The listing builds one solid part. Answer for the finished solid, in the listing's coordinates (mm). A direction names the side the tool comes from. Give positions to 0.01 mm unless a question says otherwise; leave off trailing zeros. Order: outer loops, then holes, each group sorted by start corner. A loop starts at its lowest first (then second) coordinate and runs counter-clockwise, first axis right, second up. Notation, with made-up numbers: (80, 11) - (93, 11) arc R12 cw to (93, 17) - close; hole circle Ø2 at (83.25, 16.25). An arc over 180 degrees is marked (long way). Answer in a Markdown table with one row per item. Add a question column.
Autodesk Fusion 360 part; units mm, degrees
sketch "Sketch1" plane through (0, 0, 0) normal (0, 0, 1) x (1, 0, 0)
  circle A0 centre (10, 10) radius 2.5
  line L0 (13.9, 6.1) -> (6.1, 13.9) construction
  line L1 (0, 6.4) -> (0, 1.5)
  line L2 (4.5, 1.8) -> (6.9, 1.8)
  line L3 (3.5808, 4.5) -> (6.1, 7.0192)
  line L4 (4.5, 3.5808) -> (7.0192, 6.1)
  line L5 (0.5, 6.9) -> (0.5, 6.4)
  line L6 (0.5, 6.4) -> (0, 6.4)
  line L7 (6.9, 0) -> (6.4, 0) construction
  line L8 (6.4, 0) -> (6.4, 0.5)
  line L9 (6.4, 0.5) -> (6.9, 0.5)
  arc A1 (0, 1.5) -> (1.5, 0) centre (1.5, 1.5) ccw
  line L10 (1.8, 6.9) -> (0.5, 6.9)
  line L11 (1.8, 6.9) -> (1.8, 6.4)
  line L12 (1.8, 6.4) -> (1.8, 4.5)
  line L13 (3.5808, 4.5) -> (1.8, 4.5)
  line L14 (6.1, 10) -> (6.1, 7.0192)
  line L15 (7.0192, 6.1) -> (10, 6.1)
  line L16 (4.5, 1.8) -> (4.5, 3.5808)
  line L17 (6.9, 0.5) -> (6.9, 1.8)
  line L18 (1.5, 0) -> (6.4, 0)
  line L19 (6.4, 0) -> (6.9, 0)
  line L20 (0, 6.9) -> (0, 6.4)
  line L21 (10, 13.9) -> (10, 6.1) construction
  line L22 (13.9, 10) -> (6.1, 10) construction
  line L23 (20, 6.4) -> (19.5, 6.4)
  line L24 (19.5, 6.4) -> (19.5, 6.9)
  line L25 (19.5, 6.9) -> (18.2, 6.9)
  line L26 (18.2, 4.5) -> (18.2, 6.9)
  line L27 (18.2, 4.5) -> (16.4192, 4.5)
  line L28 (16.4192, 4.5) -> (13.9, 7.0192)
  line L29 (13.9, 7.0192) -> (13.9, 10)
  line L30 (15.5, 3.5808) -> (12.9808, 6.1)
  line L31 (15.5, 3.5808) -> (15.5, 1.8)
  line L32 (13.6, 1.8) -> (15.5, 1.8)
  line L33 (13.1, 1.8) -> (13.6, 1.8)
  line L34 (13.1, 1.8) -> (13.1, 0.5)
  line L35 (13.1, 0.5) -> (13.6, 0.5)
  line L36 (13.6, 0.5) -> (13.6, 0)
  line L37 (10, 6.1) -> (12.9808, 6.1)
  line L38 (13.6, 0) -> (18.5, 0)
  arc A2 (18.5, 0) -> (20, 1.5) centre (18.5, 1.5) ccw
  line L39 (20, 1.5) -> (20, 6.4)
  line L40 (13.6, 20) -> (13.6, 19.5)
  line L41 (13.6, 19.5) -> (13.1, 19.5)
  line L42 (13.1, 19.5) -> (13.1, 18.2)
  line L43 (15.5, 18.2) -> (13.1, 18.2)
  line L44 (15.5, 18.2) -> (15.5, 16.4192)
  line L45 (15.5, 16.4192) -> (12.9808, 13.9)
  line L46 (12.9808, 13.9) -> (10, 13.9)
  line L47 (16.4192, 15.5) -> (13.9, 12.9808)
  line L48 (16.4192, 15.5) -> (18.2, 15.5)
  line L49 (18.2, 13.6) -> (18.2, 15.5)
  line L50 (18.2, 13.1) -> (18.2, 13.6)
  line L51 (18.2, 13.1) -> (19.5, 13.1)
  line L52 (19.5, 13.1) -> (19.5, 13.6)
  line L53 (19.5, 13.6) -> (20, 13.6)
  line L54 (13.9, 10) -> (13.9, 12.9808)
  line L55 (20, 13.6) -> (20, 18.5)
  arc A3 (20, 18.5) -> (18.5, 20) centre (18.5, 18.5) ccw
  line L56 (18.5, 20) -> (13.6, 20)
  line L57 (0, 13.6) -> (0.5, 13.6)
  line L58 (0.5, 13.6) -> (0.5, 13.1)
  line L59 (0.5, 13.1) -> (1.8, 13.1)
  line L60 (1.8, 15.5) -> (1.8, 13.1)
  line L61 (1.8, 15.5) -> (3.5808, 15.5)
  line L62 (3.5808, 15.5) -> (6.1, 12.9808)
  line L63 (6.1, 12.9808) -> (6.1, 10)
  line L64 (4.5, 16.4192) -> (7.0192, 13.9)
  line L65 (4.5, 16.4192) -> (4.5, 18.2)
  line L66 (6.4, 18.2) -> (4.5, 18.2)
  line L67 (6.9, 18.2) -> (6.4, 18.2)
  line L68 (6.9, 18.2) -> (6.9, 19.5)
  line L69 (6.9, 19.5) -> (6.4, 19.5)
  line L70 (6.4, 19.5) -> (6.4, 20)
  line L71 (10, 13.9) -> (7.0192, 13.9)
  line L72 (6.4, 20) -> (1.5, 20)
  arc A4 (1.5, 20) -> (0, 18.5) centre (1.5, 18.5) ccw
  line L73 (0, 18.5) -> (0, 13.6)
  arc A5 (26, 1.5) -> (27.5, 0) centre (27.5, 1.5) ccw
  line L74 (41.5, 3.5808) -> (41.5, 1.8)
  line L75 (39.1, 19.5) -> (39.1, 18.2)
  line L76 (32.4, 20) -> (27.5, 20)
  line L77 (26, 6.9) -> (26, 6.4)
  line L78 (29.5808, 4.5) -> (32.1, 7.0192)
  line L79 (29.5808, 15.5) -> (32.1, 12.9808)
  line L80 (26, 13.6) -> (26.5, 13.6)
  line L81 (39.1, 0.5) -> (39.6, 0.5)
  line L82 (30.5, 16.4192) -> (30.5, 18.2)
  line L83 (27.8, 15.5) -> (27.8, 13.1)
  line L84 (36, 13.9) -> (36, 6.1) construction
  line L85 (32.4, 0) -> (32.4, 0.5)
  line L86 (39.6, 0.5) -> (39.6, 0)
  line L87 (32.1, 10) -> (32.1, 7.0192)
  line L88 (32.4, 19.5) -> (32.4, 20)
  line L89 (39.1, 1.8) -> (39.6, 1.8)
  line L90 (27.8, 6.9) -> (27.8, 6.4)
  line L91 (41.5, 16.4192) -> (38.9808, 13.9)
  line L92 (26.5, 13.1) -> (27.8, 13.1)
  line L93 (26.5, 6.4) -> (26, 6.4)
  line L94 (32.1, 12.9808) -> (32.1, 10)
  line L95 (27.5, 0) -> (32.4, 0)
  line L96 (32.9, 0.5) -> (32.9, 1.8)
  line L97 (32.9, 0) -> (32.4, 0) construction
  line L98 (30.5, 1.8) -> (30.5, 3.5808)
  line L99 (32.9, 19.5) -> (32.4, 19.5)
  line L100 (32.9, 18.2) -> (32.4, 18.2)
  line L101 (41.5, 18.2) -> (39.1, 18.2)
  line L102 (39.6, 19.5) -> (39.1, 19.5)
  line L103 (27.8, 6.9) -> (26.5, 6.9)
  line L104 (27.8, 15.5) -> (29.5808, 15.5)
  line L105 (36, 13.9) -> (33.0192, 13.9)
  line L106 (33.0192, 6.1) -> (36, 6.1)
  line L107 (41.5, 18.2) -> (41.5, 16.4192)
  line L108 (39.9, 10) -> (32.1, 10) construction
  line L109 (39.6, 1.8) -> (41.5, 1.8)
  line L110 (39.9, 6.1) -> (32.1, 13.9) construction
  line L111 (39.6, 0) -> (44.5, 0)
  line L112 (36, 6.1) -> (38.9808, 6.1)
  circle A6 centre (36, 10) radius 2.5
  line L113 (42.4192, 4.5) -> (39.9, 7.0192)
  line L114 (38.9808, 13.9) -> (36, 13.9)
  line L115 (41.5, 3.5808) -> (38.9808, 6.1)
  line L116 (39.9, 7.0192) -> (39.9, 10)
  line L117 (39.9, 10) -> (39.9, 12.9808)
  line L118 (30.5, 16.4192) -> (33.0192, 13.9)
  line L119 (42.4192, 15.5) -> (39.9, 12.9808)
  line L120 (26, 18.5) -> (26, 13.6)
  line L121 (39.6, 20) -> (39.6, 19.5)
  line L122 (32.4, 18.2) -> (30.5, 18.2)
  line L123 (26.5, 6.9) -> (26.5, 6.4)
  line L124 (39.1, 1.8) -> (39.1, 0.5)
  arc A7 (27.5, 20) -> (26, 18.5) centre (27.5, 18.5) ccw
  line L125 (44.5, 20) -> (39.6, 20)
  line L126 (26, 6.4) -> (26, 1.5)
  line L127 (30.5, 3.5808) -> (33.0192, 6.1)
  line L128 (32.4, 0) -> (32.9, 0)
  line L129 (32.4, 0.5) -> (32.9, 0.5)
  line L130 (29.5808, 4.5) -> (27.8, 4.5)
  line L131 (27.8, 6.4) -> (27.8, 4.5)
  line L132 (30.5, 1.8) -> (32.9, 1.8)
  line L133 (26.5, 13.6) -> (26.5, 13.1)
  line L134 (32.9, 18.2) -> (32.9, 19.5)
  line L135 (59.9, 6.1) -> (52.1, 13.9) construction
  circle A8 centre (56, 10) radius 2.5
  line L136 (56, 13.9) -> (56, 6.1) construction
  line L137 (66, 13.6) -> (66, 18.5)
  line L138 (61.5, 16.4192) -> (58.9808, 13.9)
  line L139 (59.9, 10) -> (59.9, 12.9808)
  line L140 (64.2, 13.1) -> (65.5, 13.1)
  line L141 (59.6, 20) -> (59.6, 19.5)
  line L142 (52.1, 12.9808) -> (52.1, 10)
  line L143 (59.1, 19.5) -> (59.1, 18.2)
  line L144 (64.2, 13.1) -> (64.2, 13.6)
  line L145 (64.2, 13.6) -> (64.2, 15.5)
  line L146 (59.9, 10) -> (52.1, 10) construction
  line L147 (65.5, 13.1) -> (65.5, 13.6)
  line L148 (64.5, 20) -> (59.6, 20)
  line L149 (49.5808, 15.5) -> (52.1, 12.9808)
  line L150 (52.4, 19.5) -> (52.4, 20)
  line L151 (62.4192, 15.5) -> (64.2, 15.5)
  line L152 (59.1, 0.5) -> (59.6, 0.5)
  line L153 (65.5, 13.6) -> (66, 13.6)
  line L154 (50.5, 16.4192) -> (53.0192, 13.9)
  line L155 (61.5, 18.2) -> (61.5, 16.4192)
  line L156 (53.0192, 6.1) -> (56, 6.1)
  line L157 (50.5, 16.4192) -> (50.5, 18.2)
  line L158 (52.4, 0.5) -> (52.9, 0.5)
  line L159 (59.1, 1.8) -> (59.6, 1.8)
  line L160 (49.5808, 4.5) -> (52.1, 7.0192)
  line L161 (50.5, 1.8) -> (50.5, 3.5808)
  line L162 (61.5, 3.5808) -> (61.5, 1.8)
  line L163 (56, 13.9) -> (53.0192, 13.9)
  line L164 (52.4, 0) -> (52.4, 0.5)
  line L165 (50.5, 3.5808) -> (53.0192, 6.1)
  line L166 (66, 1.5) -> (66, 6.4)
  line L167 (59.6, 1.8) -> (61.5, 1.8)
  arc A9 (66, 18.5) -> (64.5, 20) centre (64.5, 18.5) ccw
  line L168 (52.1, 10) -> (52.1, 7.0192)
  line L169 (64.2, 4.5) -> (62.4192, 4.5)
  line L170 (59.6, 19.5) -> (59.1, 19.5)
  line L171 (61.5, 18.2) -> (59.1, 18.2)
  line L172 (61.5, 3.5808) -> (58.9808, 6.1)
  line L173 (52.9, 0) -> (52.4, 0) construction
  line L174 (59.9, 7.0192) -> (59.9, 10)
  line L175 (52.4, 18.2) -> (50.5, 18.2)
  line L176 (59.6, 0.5) -> (59.6, 0)
  line L177 (52.9, 18.2) -> (52.4, 18.2)
  line L178 (66, 6.4) -> (65.5, 6.4)
  line L179 (56, 6.1) -> (58.9808, 6.1)
  line L180 (52.9, 18.2) -> (52.9, 19.5)
  line L181 (59.6, 0) -> (64.5, 0)
  line L182 (62.4192, 4.5) -> (59.9, 7.0192)
  arc A10 (64.5, 0) -> (66, 1.5) centre (64.5, 1.5) ccw
  line L183 (50.5, 1.8) -> (52.9, 1.8)
  line L184 (52.4, 20) -> (47.5, 20)
  line L185 (64.2, 4.5) -> (64.2, 6.9)
  line L186 (65.5, 6.4) -> (65.5, 6.9)
  line L187 (52.4, 0) -> (52.9, 0)
  line L188 (52.9, 19.5) -> (52.4, 19.5)
  line L189 (65.5, 6.9) -> (64.2, 6.9)
  line L190 (59.1, 1.8) -> (59.1, 0.5)
  line L191 (47.5, 0) -> (52.4, 0)
  line L192 (58.9808, 13.9) -> (56, 13.9)
  line L193 (62.4192, 15.5) -> (59.9, 12.9808)
  line L194 (52.9, 0.5) -> (52.9, 1.8)
  line L195 (44.5, 20) -> (47.5, 20)
  line L196 (44.5, 0) -> (47.5, 0)
  line L197 (41.5, 18.2) -> (42.8, 18.2) construction
  line L198 (42.8, 18.2) -> (49.2, 18.2)
  line L199 (49.2, 1.8) -> (42.8, 1.8)
  line L200 (42.4192, 15.5) -> (42.8, 15.8808)
  line L201 (49.5808, 15.5) -> (49.2, 15.8808)
  line L202 (49.5808, 4.5) -> (49.2, 4.1192)
  line L203 (42.4192, 4.5) -> (42.8, 4.1192)
  line L204 (42.8, 15.8808) -> (42.8, 18.2)
  line L205 (49.2, 18.2) -> (49.2, 15.8808)
  line L206 (49.2, 4.1192) -> (49.2, 1.8)
  line L207 (42.8, 1.8) -> (42.8, 4.1192)
  point P0 (10, 10)
  point P1 (36, 10)
  point P2 (56, 10)
  dimension "d3" = 5
  dimension "d6" = 6.9
  dimension "d7" = 6.9
  dimension "d14" = 6.4
  dimension "d22" = 0.5
  dimension "d23" = 0.5
  dimension "d24" = 0.5
  dimension "d25" = 0.5
  dimension "d26" = 1.5
  dimension "d28" = 360
  dimension "d30" = 360
  dimension "d31" = 5
  dimension "d32" = 0.5
  dimension "d33" = 0.5
  dimension "d34" = 0.5
  dimension "d35" = 0.5
  dimension "d36" = 1.5
  dimension "d39" = 5
  dimension "d42" = 0.5
  dimension "d43" = 0.5
  dimension "d45" = 1.3
  dimension "d47" = 6.4
extrude "Extrude1" add sketch "Sketch1" along normal blind 100 makes body 1 at (12.4876, 9.7511, 33.3333) makes body 2 at (38.4876, 9.7511, 33.3333)
hidden bodies 2
equation "d7 = 10 mm - 3.1 mm"
equation "d14 = 10 mm - 3.6 mm"
(1) Find section A-A, the plane x = 10. Write down the section's boundary in (y, z).
(2) Each of these flat-tipped pins is pushed along its axis until it touches: P1, Ø2, axis at x = 9, z = 66.5, coming from the +Y side; P2, Ø4, axis at y = 18, z = 60, coming from the -X side; P3, Ø0.6, axis at x = 20, z = 61.5, coming from the -Y side; P4, Ø2, axis at x = 14, y = 17, coming from the +Z side. Where does it stop, or does it pass through?
(3) For faces 4 (the face through (14.26, 4.82, 49.3)), 5 (the face through (20, 16, 49)), determine the directions among +Z, -Z, +X, -X, +Y, -Y from which every point of the face is accessible in a straight line to the end or side of a thin tool.
(4) The mould has two halves that part along X. Classify faces 1 (the face through (8, 12, 100)), 2 (the face through (13.9, 10, 49)), 3 (the face through (6, 1.8, 49)): +X half, -X half, draft (parallel to the pull), parting line (faces both ways), or undercut.
(5) Straight lines are drawn through the part: line 1 (X direction, y = 18.75, z = 57); line 2 (Y direction, x = 10, z = 45.5); line 3 (Y direction, x = 2.25, z = 91). For each, find the intervals that lie inside material, in ascending order.
Answer key:
| question | item | result |
|---|---|---|
| 1 | outline | (6.1, 0) - (7.5, 0) - (7.5, 100) - (6.1, 100) - close; (12.5, 0) - (13.9, 0) - (13.9, 100) - (12.5, 100) - close |
| 2 | P1 | y = 13.9 |
| 2 | P2 | x = 0 |
| 2 | P3 | y = 0.6 |
| 2 | P4 | through |
| 3 | face 4 | +Z, -Z |
| 3 | face 5 | +Z, -Z, +X, +Y, -Y |
| 4 | face 1 | draft |
| 4 | face 2 | +X half |
| 4 | face 3 | undercut |
| 5 | line 1 | 0.02 to 6.9, 13.1 to 19.98 |
| 5 | line 2 | 6.1 to 7.5, 12.5 to 13.9 |
| 5 | line 3 | 0 to 4.5, 15.5 to 20 |
